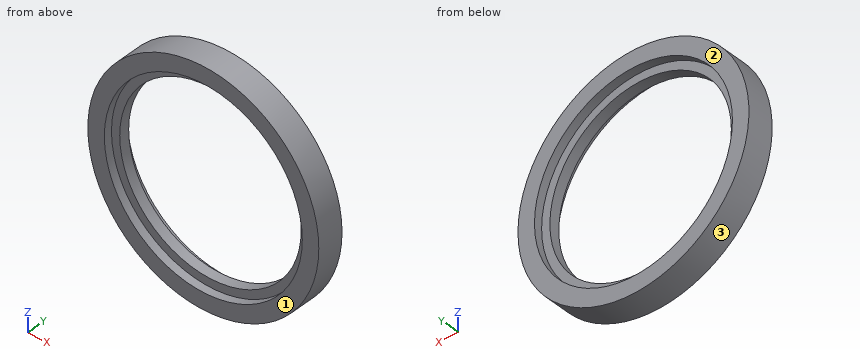
Autodesk Inventor part; units mm, degrees
ref_plane "YZ Plane" through (0, 0, 0) normal (1, 0, 0) x (0, 1, 0)
ref_plane "XZ Plane" through (0, 0, 0) normal (0, 1, 0) x (-1, 0, 0)
ref_plane "XY Plane" through (0, 0, 0) normal (0, 0, 1) x (1, 0, 0)
sketch "Boceto1" plane through (0, 0, 0) normal (0, 0, 1) x (1, 0, 0)
  line L0 (0, 0) -> (56, 0) construction
  line L1 (56, 0) -> (56, 13)
  line L2 (56, 13) -> (48, 13)
  line L3 (48, 13) -> (48, 9)
  line L4 (48, 9) -> (44, 9)
  line L5 (44, 9) -> (44, 4)
  line L6 (44, 4) -> (48, 4)
  line L7 (48, 4) -> (48, 0)
  line L8 (48, 0) -> (56, 0)
  line L9 (0, 0) -> (0, 24.3321) construction
  dimension "d0" = 56
  dimension "d1" = 13
  dimension "d2" = 8
  dimension "d3" = 4
  dimension "d4" = 4
  dimension "d5" = 5
  dimension "d6" = 4
revolve "Revolución1" add sketch "Boceto1" angle 360 about axis through (0, 0, 0) along (0, 1, 0)
properties part number "20_AnilloPorSoldar2"
For this review, take the finished solid that the model builds, in its own axes (mm). Face numbers are marked on the shaded views. Coordinates: 2 decimals unless noted, no trailing zeros. Write each loop counter-clockwise with the first axis right and the second up, starting at its lowest first coordinate (ties: lowest second). Pieces come first, ordered by that corner, then holes. Notation, with made-up numbers: (-21.75, -23) -> (20.25, -23) arc R16 ccw to (20.25, -3) -> close; hole circle Ø3 at (33, 20.5). An arc over 180 degrees is marked (long way). Write each question's results on one line, items separated by ' | '. Start each with the question number.
1) Wall thickness on L1, parallel to Z at x = 0, y = 1.25; L2, parallel to Z at x = 0, y = 5.55: over which ranges is each line inside the solid? List them lowest first. Write a range as [from, to].
2) Consider section A-A (x = 0). Write out the cut boundary in (y, z).
3) The part is to be moulded in two halves that separate along Y. For the marked faces 1, 2 and 3, say which applies: +Y half, -Y half, draft (parallel to the pull), parting line (faces both ways), or undercut.
4) Insertion check: pin 1 (2 mm diameter, centred on y = 3, z = 17.5, fed in from -X); pin 2 (3 mm diameter, centred on y = 9, z = 25, fed in from +X); pin 3 (12 mm diameter, centred on x = -35, z = -32.5, fed in from +Y); pin 4 (3 mm diameter, centred on y = 10, z = -26, fed in from -X). Each pin has a flat end and moves straight along its axis. Give the tip position at first contact, or say it passes through.
5) Consider section C-C (y = 11.25). Write out the cut boundary in (x, z), plus the area to 3 significant figures.
6) Consider section B-B (z = 33). Write out the cut boundary in (x, y), plus the area to 3 significant figures.
Geometry says:
1) L1: [-56, -48], [48, 56] | L2: [-56, -44], [44, 56]
2) outline: (0, -56) -> (13, -56) -> (13, -48) -> (9, -48) -> (9, -44) -> (4, -44) -> (4, -48) -> (0, -48) -> close; (0, 48) -> (4, 48) -> (4, 44) -> (9, 44) -> (9, 48) -> (13, 48) -> (13, 56) -> (0, 56) -> close
3) face 1: -Y half | face 2: +Y half | face 3: draft
4) pin 1: x = -53.51 | pin 2: x = 50.83 | pin 3: y = 13 | pin 4: x = -50.36
5) outline: circle Ø112 at (0, 0); hole circle Ø96 at (0, 0) | area: 2,610 mm^2
6) outline: (-45.24, 0) -> (-34.86, 0) -> (-34.86, 4) -> (-29.1, 4) -> (-29.1, 9) -> (-34.86, 9) -> (-34.86, 13) -> (-45.24, 13) -> close; (29.1, 4) -> (34.86, 4) -> (34.86, 0) -> (45.24, 0) -> (45.24, 13) -> (34.86, 13) -> (34.86, 9) -> (29.1, 9) -> close | area: 328 mm^2
